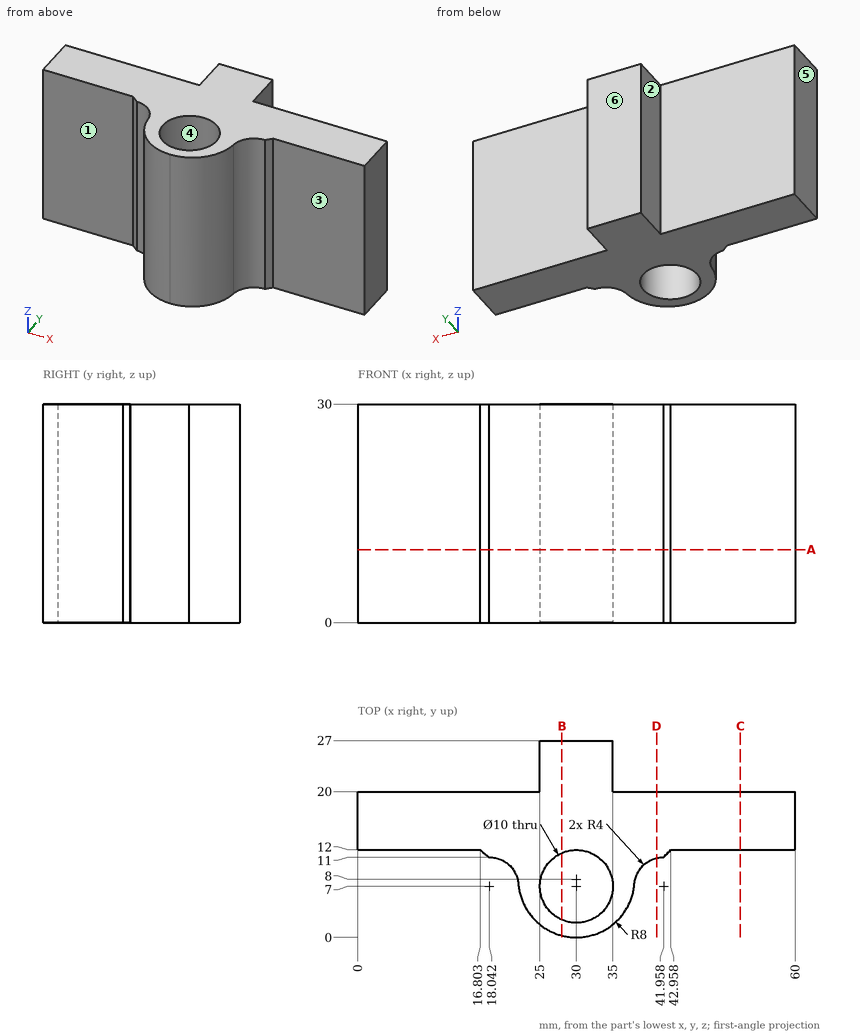
The figure shows three views and two pictorial views of one solid part (mm, origin at its lowest corner). Answer the questions. A direction names the side the tool comes from. Coordinates: 2 decimals unless noted, no trailing zeros. Loops run counter-clockwise (first coordinate to the right, second up) from the corner with the lowest first, then second, coordinate; pieces in that order, holes last. Notation, with made-up numbers: (86.25, 76) - (126.25, 76) arc R14 cw to (126.25, 91) - close; hole circle Ø4 at (-32.5, 16). An arc over 180 degrees is marked (long way). Answer in a Markdown table with one row per item.
Q1. Find section A-A on z = 10. Write down the section's boundary in (x, y).
Here are the results:
| item | result |
|---|---|
| outline | (0, 12) - (16.8, 12) - (18.04, 11) arc R4 cw to (22.03, 7.33) arc R8 ccw to (37.97, 7.33) arc R4 cw to (41.96, 11) - (42.96, 12) - (60, 12) - (60, 20) - (35, 20) - (35, 27) - (25, 27) - (25, 20) - (0, 20) - close; hole circle Ø10 at (30, 7) |
Q2. For the marked faces 1, 2 and 3, determine the directions among +Z, -Z, +X, -X, +Y, -Y from which every point of the face is accessible in a straight line to the end or side of a thin tool.
Here are the results:
| item | result |
|---|---|
| face 1 | +Z, -Z, -X, -Y |
| face 2 | +Z, -Z, -X, +Y |
| face 3 | +Z, -Z, +X, -Y |
Q3. Given P1, Ø1.5, axis at y = 4.5, z = 24, coming from the +X side; P2, Ø1, axis at x = 41.5, z = 16, coming from the -Y side; P3, Ø7.5, axis at x = 42, z = 10.5, coming from the +Y side, each flat-ended and moving along its own axis, determine where each tip first touches the part or whether it passes through.
Here are the results:
| item | result |
|---|---|
| P1 | stops at x = 37.51 |
| P2 | stops at y = 10.88 |
| P3 | stops at y = 20 |
Q4. Straight lines are drawn through the part: line 1 along Y through (x, z) = (30, 7); line 2 along X through (y, z) = (7.25, 2) (1 decimal); line 3 along Y through (x, z) = (55.5, 9.25). For each, find the intervals that lie inside material, in ascending order. Write a range as [from, to].
Here are the results:
| item | result |
|---|---|
| line 1 | y = [0, 2], [12, 27] |
| line 2 | x = [22, 25], [35, 38] |
| line 3 | y = [12, 20] |
Q5. Find section C-C on x = 52.5. Write down the section's boundary in (y, z), plus the area to 3 significant figures.
Here are the results:
| item | result |
|---|---|
| outline | (12, 0) - (20, 0) - (20, 30) - (12, 30) - close |
| area | 240 mm^2 |
Q6. Find section D-D on x = 41. Write down the section's boundary in (y, z).
Here are the results:
| item | result |
|---|---|
| outline | (10.88, 0) - (20, 0) - (20, 30) - (10.88, 30) - close |
Q7. Find section B-B on x = 28. Write down the section's boundary in (y, z).
Here are the results:
| item | result |
|---|---|
| outline | (0.25, 0) - (2.42, 0) - (2.42, 30) - (0.25, 30) - close; (11.58, 0) - (27, 0) - (27, 30) - (11.58, 30) - close |
Q8. The mould has two halves that part along X. Classify the marked faces 4, 5 and 6: pulls with the +X half, pulls with the -X half, needs draft (parallel to the pull), parting line crosses it, or undercut.
Here are the results:
| item | result |
|---|---|
| face 4 | undercut |
| face 5 | pulls with the -X half |
| face 6 | needs draft |
